from build123d import *

# Parameters (mm, degrees)
ESQUISSE2_R        = 1.6
ESQUISSE2_R_2      = 57.25
BOSS_EXTRU_2_DEPTH = 5


with BuildPart() as part:
    # Esquisse2 → Boss.-Extru.2 (new body)
    with BuildSketch(Plane.XY):
        with BuildLine():
            Line((-21.972994789, 62.5), (21.972994789, 62.5))
            ThreePointArc((21.972994789, 62.5), (66.25, 0), (21.972994789, -62.5))
            Line((21.972994789, -62.5), (-21.972994789, -62.5))
            ThreePointArc((-21.972994789, -62.5), (-66.25, 0), (-21.972994789, 62.5))
        make_face()
        with Locations((60, 19)):
            Circle(ESQUISSE2_R, mode=Mode.SUBTRACT)
        with Locations((60, -19)):
            Circle(ESQUISSE2_R, mode=Mode.SUBTRACT)
        with Locations((-60, -19)):
            Circle(ESQUISSE2_R, mode=Mode.SUBTRACT)
        with Locations((-60, 19)):
            Circle(ESQUISSE2_R, mode=Mode.SUBTRACT)
        Circle(ESQUISSE2_R_2, mode=Mode.SUBTRACT)
    extrude(amount=BOSS_EXTRU_2_DEPTH)


solid = part.part
Part model, mm, in its own coordinate system. Round coordinates to 2 decimals unless told otherwise and drop trailing zeros. Write each loop counter-clockwise with the first axis right and the second up, starting at its lowest first coordinate (ties: lowest second). Pieces come first, ordered by that corner, then holes. Notation, with made-up numbers: M 57.5,64 L 70.5,64 A13 ccw 70.5,74 Z; hole C 59,33 d5. An arc over 180 degrees is marked long. Return JSON: item names as keys, results as strings. Group by question number.
(1) Saw through at C-C on z = 2.85. Write the cut outline in (x, y).
(2) Pin check, flat tips, straight feed: pin 1 Ø2 at (x, z) = (-27.5, 1) entering from +Y; pin 2 Ø3 at (x, y) = (60, 19) entering from +Z. Stop position of each tip, or through.
(3) Saw through at D-D on x = -17.5. Write the cut outline in (y, z).
(4) Two-plate mould, pull along X, no slides. Class faces 1 (the face through (-66.24, -1.14, 2.46)), 2 (the face through (40, 42, 5)), 3 (the face through (60.86, 20.35, 2.46)): +X half, -X half, draft (parallel to the pull), parting line (faces both ways), or undercut.
(5) Drill centre lines: probe 1 along Y at (x, z) = (0, 1.3); probe 2 along Y at (x, z) = (-61, 3.3); probe 3 along Y at (x, z) = (60, 3.3). Where is each one in solid material? Low to high.
(6) Saw through at A-A on y = 0. Write the cut outline in (x, z).
(7) Saw through at B-B on x = -60. Write the cut outline in (y, z).
Returned:
{
 "1": {"outline": "M -21.97,-62.5 L 21.97,-62.5 A66.25 ccw 21.97,62.5 L -21.97,62.5 A66.25 ccw Z; hole C -60,-19 d3.2; hole C -60,19 d3.2; hole C 0,0 d114.5; hole C 60,-19 d3.2; hole C 60,19 d3.2"},
 "2": {"pin 1": "y = 60.72", "pin 2": "through"},
 "3": {"outline": "M -62.5,0 L -54.51,0 L -54.51,5 L -62.5,5 Z; M 54.51,0 L 62.5,0 L 62.5,5 L 54.51,5 Z"},
 "4": {"face 1": "-X half", "face 2": "draft", "face 3": "undercut"},
 "5": {"probe 1": "-62.5 to -57.25, 57.25 to 62.5", "probe 2": "-25.85 to -20.25, -17.75 to 17.75, 20.25 to 25.85", "probe 3": "-28.09 to -20.6, -17.4 to 17.4, 20.6 to 28.09"},
 "6": {"outline": "M -66.25,0 L -57.25,0 L -57.25,5 L -66.25,5 Z; M 57.25,0 L 66.25,0 L 66.25,5 L 57.25,5 Z"},
 "7": {"outline": "M -28.09,0 L -20.6,0 L -20.6,5 L -28.09,5 Z; M -17.4,0 L 17.4,0 L 17.4,5 L -17.4,5 Z; M 20.6,0 L 28.09,0 L 28.09,5 L 20.6,5 Z"}
}
